Design review of the part built by this model. Coordinates are the model's own, in mm. Face numbers are marked on the shaded views. A direction names the side the tool comes from. Give positions to 0.01 mm unless a question says otherwise; leave off trailing zeros. Loops run counter-clockwise (first coordinate to the right, second up) from the corner with the lowest first, then second, coordinate; pieces in that order, holes last. Notation, with made-up numbers: M 1.25,75 L 40.25,75 A25 ccw 40.25,111 Z; hole C 8.5,57 d2. An arc over 180 degrees is marked long. Answer as CSV lines item,"result".
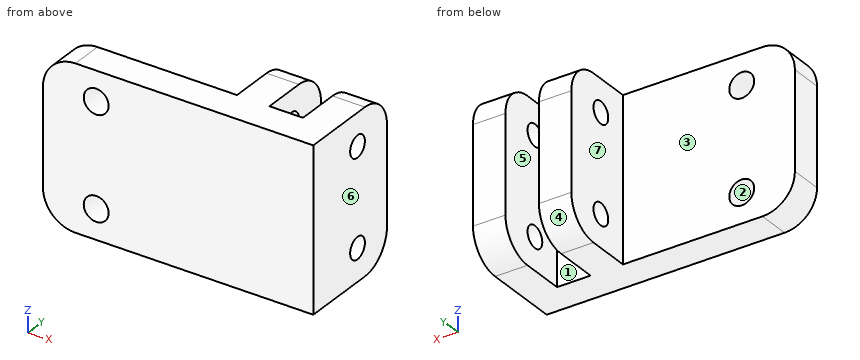
```python
from build123d import *

# Parameters (mm, degrees)
SKETCH1_W               = 15.9
SKETCH1_H               = 15
SKETCH1_R               = 1.15
SKETCH1_W_2             = 3
SKETCH1_W_3             = 3.1
BOSS_EXTRUDE1_DEPTH     = 3
FILLET1_R               = 3
SKETCH1_3_W             = 3
SKETCH1_3_H             = 15
BOSS_EXTRUDE2_DEPTH     = 10
CUT_EXTRUDE1_DEPTH      = 25.037678756
CUT_EXTRUDE1_DEPTH_BACK = 25.037678756
SKETCH2_R               = 1
FILLET2_R               = 3


with BuildPart() as part:
    # Sketch1 → Boss-Extrude1 (new body)
    # profile 1 of 4: a face of its own
    with BuildSketch(Plane(origin=(0, 0, 0), x_dir=(1, 0, 0), z_dir=(0, 1, 0))):
        with Locations((7.95, 7.5)):
            Rectangle(SKETCH1_W, SKETCH1_H)
        with Locations(Location((4.917465758, 2.75, 0), (0, 0, 270))):
            Circle(SKETCH1_R, mode=Mode.SUBTRACT)
        with Locations(Location((4.917465758, 12.25, 0), (0, 0, 270))):
            Circle(SKETCH1_R, mode=Mode.SUBTRACT)
    # profile 2 of 4: a face of its own
    with BuildSketch(Plane(origin=(0, 0, 0), x_dir=(1, 0, 0), z_dir=(0, 1, 0))):
        with Locations((17.4, 7.5)):
            Rectangle(SKETCH1_W_2, SKETCH1_H)
    # profile 3 of 4: a face of its own
    with BuildSketch(Plane(origin=(0, 0, 0), x_dir=(1, 0, 0), z_dir=(0, 1, 0))):
        with Locations((20.45, 7.5)):
            Rectangle(SKETCH1_W_3, SKETCH1_H)
    # profile 4 of 4: a face of its own
    with BuildSketch(Plane(origin=(0, 0, 0), x_dir=(1, 0, 0), z_dir=(0, 1, 0))):
        with Locations((23.5, 7.5)):
            Rectangle(SKETCH1_W_2, SKETCH1_H)
    extrude(amount=BOSS_EXTRUDE1_DEPTH)

    # Fillet1
    fillet1_edges = [part.edges().sort_by_distance(p)[0] for p in [
        (0, 1.5, 0),
        (0, 1.5, -15),
        (25, 1.5, -15),
        (25, 1.5, 0),
    ]]
    fillet(fillet1_edges, radius=FILLET1_R)

    # Sketch1_3 → Boss-Extrude2 (add)
    with BuildSketch(Plane(origin=(0, 0, 0), x_dir=(1, 0, 0), z_dir=(0, 1, 0))):
        with Locations((17.4, 7.5)):
            Rectangle(SKETCH1_3_W, SKETCH1_3_H)
        with Locations((23.5, 7.5)):
            Rectangle(SKETCH1_3_W, SKETCH1_3_H)
    extrude(amount=BOSS_EXTRUDE2_DEPTH)

    # Sketch2 → Cut-Extrude1 (cut, two sides: drawn at the far end of the back side and taken through both)
    with BuildSketch(Plane.ZY.offset(-15.9).offset(-CUT_EXTRUDE1_DEPTH_BACK)):
        with Locations((-12, 6)):
            Circle(SKETCH2_R)
        with Locations((-3, 6)):
            Circle(SKETCH2_R)
    extrude(amount=CUT_EXTRUDE1_DEPTH + CUT_EXTRUDE1_DEPTH_BACK, mode=Mode.SUBTRACT)

    # Fillet2
    fillet2_edges = [part.edges().sort_by_distance(p)[0] for p in [
        (17.4, 10, -15),
        (17.4, 10, 0),
        (23.5, 10, -15),
        (23.5, 10, 0),
    ]]
    fillet(fillet2_edges, radius=FILLET2_R)


solid = part.part
```
1. For P1, Ø3, axis at y = 6.5, z = -9.5, coming from the -X side; P2, Ø1.5, axis at x = 5.5, z = -5.5, coming from the +Y side, all flat-tipped, find the tip position at first contact; note any pin that passes through.
Answer block:
P1,"x = 15.9"
P2,"y = 3"
2. We need section B-B, the plane y = 6. Write out the cut boundary in (x, z).
Answer block:
outline,"M 15.9,-15 L 18.9,-15 L 18.9,-13 L 15.9,-13 Z; M 15.9,-11 L 18.9,-11 L 18.9,-4 L 15.9,-4 Z; M 15.9,-2 L 18.9,-2 L 18.9,0 L 15.9,0 Z; M 22,-15 L 25,-15 L 25,-13 L 22,-13 Z; M 22,-11 L 25,-11 L 25,-4 L 22,-4 Z; M 22,-2 L 25,-2 L 25,0 L 22,0 Z"
3. We need section D-D, the plane z = -9.5. Write out the cut boundary in (x, y).
Answer block:
outline,"M 0,0 L 25,0 L 25,10 L 22,10 L 22,3 L 18.9,3 L 18.9,10 L 15.9,10 L 15.9,3 L 0,3 Z"
4. To check wall thickness, follow L1, parallel to Z at x = 17.3, y = 6; L2, parallel to X at y = 6.75, z = -4; L3, parallel to Y at x = 21, z = -9.75. State the ranges of each line that lie inside material, in increasing order. Write a range as [from, to].
Answer block:
L1,"[-15, -13], [-11, -4], [-2, 0]"
L2,"[15.9, 18.9], [22, 25]"
L3,"[0, 3]"
5. We need section C-C, the plane z = -2.75. Write out the cut boundary in (x, y), plus the area to 3 significant figures.
Answer block:
outline,"M 0.01,0 L 3.77,0 L 3.77,3 L 0.01,3 Z; M 6.07,0 L 25,0 L 25,5.03 L 22,5.03 L 22,3 L 18.9,3 L 18.9,5.03 L 15.9,5.03 L 15.9,3 L 6.07,3 Z; M 15.9,6.97 L 18.9,6.97 L 18.9,9.99 L 15.9,9.99 Z; M 22,6.97 L 25,6.97 L 25,9.99 L 22,9.99 Z"
area,"98.4 mm²"
6. We need section A-A, the plane y = 4.25. Write out the cut boundary in (x, z), plus the area to 3 significant figures.
Answer block:
outline,"M 15.9,-15 L 18.9,-15 L 18.9,0 L 15.9,0 Z; M 22,-15 L 25,-15 L 25,0 L 22,0 Z"
area,"90.0 mm²"
7. The part is to be moulded in two halves that separate along X. For the marked faces 4, 5, 6 and 7, say which applies: pulls with the +X half, pulls with the -X half, needs draft (parallel to the pull), parting line crosses it, or undercut.
Answer block:
face 4,"needs draft"
face 5,"undercut"
face 6,"pulls with the +X half"
face 7,"pulls with the -X half"
8. For the marked faces 1, 2 and 3, list the 3-axis set-ups (+Z, -Z, +X, -X, +Y, -Y) from which the entire face can be reached by the end or side of a thin tool; tool diameter is ignored.
Answer block:
face 1,"+Z, -Z, +Y"
face 2,"+Y, -Y"
face 3,"+Z, -Z, -X, +Y"
